For this review, take the finished solid that the model builds, in its own axes (mm). A direction names the side the tool comes from. Coordinates: 2 decimals unless noted, no trailing zeros. Loops run counter-clockwise (first coordinate to the right, second up) from the corner with the lowest first, then second, coordinate; pieces in that order, holes last.
1. Take a section at B-B, the plane y = -24. State the section outline as (x, z) points.
2. Take a section at C-C, the plane y = 5. State the section outline as (x, z) points.
3. Clearance check with flat-ended pins moving along their axes: P1, Ø12, axis at y = 19, z = -8.5, coming from the +X side; P2, Ø12, axis at x = -5.5, z = -12.5, coming from the +Y side; P3, Ø6.5, axis at x = 0, z = -19.5, coming from the -Y side. State where each tip first meets the part, or that it passes through.
4. Take a section at A-A, the plane x = 13. State the section outline as (y, z) points.
5. To check wall thickness, follow probe 1 along X at (y, z) = (14.5, -13.5); probe 2 along Z at (x, y) = (2.5, 20.5); probe 3 along Z at (x, y) = (-11.5, -7.5). State the ranges of each line that lie inside material, in increasing order.
6. Take a section at D-D, the plane z = -11.5. State the section outline as (x, y) points.
7. Machinability: for faces 1 (the face through (-9.639, 0, 10)), 2 (the face through (0, 21.946, -17)), 3 (the face through (0, -21.946, -17)), 4 (the face through (10.732, 0, -17)), which of the approach directions +Z, -Z, +X, -X, +Y, -Y give a long, thin tool a straight path to every point of the face, cutting with its end or side? Answer none if there is none.
```python
from build123d import *

# Parameters (mm, degrees)
SKETCH1_W           = 33.4264
SKETCH1_H           = 56.8452
BOSS_EXTRUDE1_DEPTH = 2.54
SKETCH2_W           = 27.6352
SKETCH2_H           = 50.6984
BOSS_EXTRUDE2_DEPTH = 3.048
SKETCH3_W           = 19.2786
SKETCH3_H           = 37.1856
BOSS_EXTRUDE3_DEPTH = 9.0424
FILLET1_R           = 2.54
FILLET7_R           = 8.636
SKETCH4_W           = 21.463
SKETCH4_H           = 43.8912
BOSS_EXTRUDE4_DEPTH = 34.0868


with BuildPart() as part:
    # Sketch1 → Boss-Extrude1 (new body)
    with BuildSketch(Plane.XY):
        Rectangle(SKETCH1_W, SKETCH1_H)
    extrude(amount=BOSS_EXTRUDE1_DEPTH)

    # Sketch2 → Boss-Extrude2 (add)
    with BuildSketch(Plane.XY.offset(2.54)):
        Rectangle(SKETCH2_W, SKETCH2_H)
    extrude(amount=BOSS_EXTRUDE2_DEPTH)

    # Sketch3 → Boss-Extrude3 (add)
    with BuildSketch(Plane.XY.offset(5.588)):
        Rectangle(SKETCH3_W, SKETCH3_H)
    extrude(amount=BOSS_EXTRUDE3_DEPTH)

    # Fillet1
    fillet1_edges = [part.edges().sort_by_distance(p)[0] for p in [
        (13.8176, 0, 2.54),
        (0, 25.3492, 2.54),
        (-13.8176, 0, 2.54),
        (0, -25.3492, 2.54),
    ]]
    fillet(fillet1_edges, radius=FILLET1_R)

    # Fillet7
    fillet7_edges = [part.edges().sort_by_distance(p)[0] for p in [
        (0, 18.5928, 14.6304),
        (0, -18.5928, 14.6304),
    ]]
    fillet(fillet7_edges, radius=FILLET7_R)

    # Sketch4 → Boss-Extrude4 (add)
    with BuildSketch(Plane(origin=(0, 0, 0), x_dir=(-1, 0, 0), z_dir=(0, 0, -1))):
        Rectangle(SKETCH4_W, SKETCH4_H)
    extrude(amount=BOSS_EXTRUDE4_DEPTH)


solid = part.part
```
Results list:
1. outline: (-16.71, 0) - (16.71, 0) - (16.71, 2.54) - (16.36, 2.54) arc R2.54 cw to (13.82, 5.08) - (13.82, 5.59) - (-13.82, 5.59) - (-13.82, 5.08) arc R2.54 cw to (-16.36, 2.54) - (-16.71, 2.54) - close
2. outline: (-16.71, 0) - (-10.73, 0) - (-10.73, -34.09) - (10.73, -34.09) - (10.73, 0) - (16.71, 0) - (16.71, 2.54) - (16.36, 2.54) arc R2.54 cw to (13.82, 5.08) - (13.82, 5.59) - (9.64, 5.59) - (9.64, 14.63) - (-9.64, 14.63) - (-9.64, 5.59) - (-13.82, 5.59) - (-13.82, 5.08) arc R2.54 cw to (-16.36, 2.54) - (-16.71, 2.54) - close
3. P1: stops at x = 10.73
3. P2: stops at y = 21.95
3. P3: stops at y = -21.95
4. outline: (-28.42, 0) - (28.42, 0) - (28.42, 2.54) - (27.89, 2.54) arc R2.54 cw to (25.35, 5.08) - (25.35, 5.59) - (-25.35, 5.59) - (-25.35, 5.08) arc R2.54 cw to (-27.89, 2.54) - (-28.42, 2.54) - close
5. probe 1: x = -10.73 to 10.73
5. probe 2: z = -34.09 to 5.59
5. probe 3: z = 0 to 5.59
6. outline: (-10.73, -21.95) - (10.73, -21.95) - (10.73, 21.95) - (-10.73, 21.95) - close
7. face 1: +Z, -X, +Y, -Y
7. face 2: -Z, +X, -X, +Y
7. face 3: -Z, +X, -X, -Y
7. face 4: -Z, +X, +Y, -Y
